Could you check a few things on this model? Use its own coordinates, in mm. Face numbers are marked on the shaded views. Give positions to 0.01 mm unless a question says otherwise; leave off trailing zeros. Loops run counter-clockwise (first coordinate to the right, second up) from the corner with the lowest first, then second, coordinate; pieces in that order, holes last. Notation, with made-up numbers: M 75.25,55.5 L 98.25,55.5 A25 ccw 98.25,72.5 Z; hole C 54.5,80 d4. An arc over 180 degrees is marked long. Write each question's results on one line, items separated by ' | '. Start each with the question number.
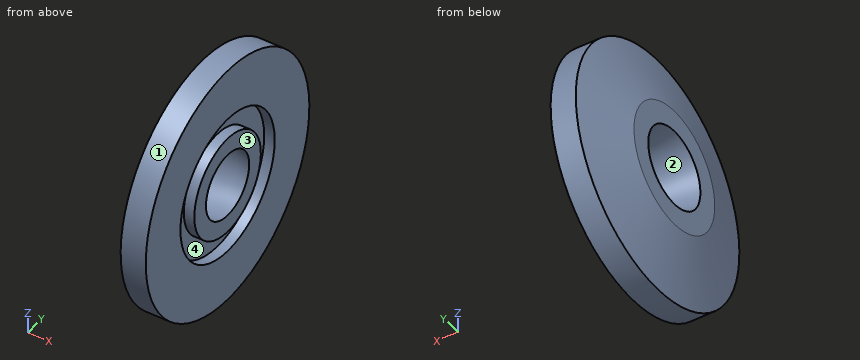
from build123d import *


with BuildPart() as part:
    # Sketch1 → Revolve1 (revolve)
    with BuildSketch(Plane.XY, mode=Mode.PRIVATE) as revolve1_sk:
        Polygon((-2.54, 8.636), (-2.54, 14.986), (-5.588, 14.986), (-7.62, 7.402472759), (-7.62, 0), (-2.54, 0), (-2.54, 6.096), (-3.81, 6.096), (-3.81, 8.636), align=None)
    revolve(revolve1_sk.sketch.rotate(Axis((-12.512764007, 0, 0), (-1, 0, 0)), 90), axis=Axis((-12.512764007, 0, 0), (-1, 0, 0)))

    # Sketch2 → Cut-Revolve1 (revolve, cut)
    with BuildSketch(Plane.XY, mode=Mode.PRIVATE) as cut_revolve1_sk:
        Polygon((-9.728542139, 0), (0.013390026, 0), (0.013390026, 3.553074477), (-9.728542139, 5.111363938), align=None)
    revolve(cut_revolve1_sk.sketch.rotate(Axis((-9.728542139, 0, 0), (-1, 0, 0)), 270), axis=Axis((-9.728542139, 0, 0), (-1, 0, 0)), mode=Mode.SUBTRACT)


solid = part.part
1) Thinking about a two-plate mould opening in Y: for the marked faces 1, 2, 3 and 4, which applies, pulls with the +Y half, pulls with the -Y half, needs draft (parallel to the pull), parting line crosses it, or undercut?
2) If we section it at A-A on y = 0: Write out the boundary of the cut face in (x, z), plus the area to 3 significant figures.
3) If we section it at C-C on x = -6.9: Write out the boundary of the cut face in (y, z).
4) I'm going to push flat-ended pins straight in: P1, Ø1.5, axis at y = -7, z = 1, coming from the +X side; P2, Ø2, axis at y = -8, z = 3, coming from the +X side. Where does each tip first touch, or does it pass through?
5) Please list where these lines run through material, in increasing order: line 1 (Y direction, x = -3.1, z = 0); line 2 (Y direction, x = -3.25, z = 0); line 3 (Y direction, x = -3, z = 4.25). Write a range as from..to.
Calculated:
1) face 1: parting line crosses it | face 2: undercut | face 3: needs draft | face 4: undercut
2) outline: M -7.62,-7.4 L -5.59,-14.99 L -2.54,-14.99 L -2.54,-8.64 L -3.81,-8.64 L -3.81,-6.1 L -2.54,-6.1 L -2.54,-3.96 L -7.62,-4.77 Z; M -7.62,4.77 L -2.54,3.96 L -2.54,6.1 L -3.81,6.1 L -3.81,8.64 L -2.54,8.64 L -2.54,14.99 L -5.59,14.99 L -7.62,7.4 Z | area: 86.0 mm2
3) outline: C 0,0 d20.18; hole C 0,0 d9.32
4) P1: stops at x = -3.81 | P2: stops at x = -2.54
5) line 1: y = -14.99..-8.64, -6.1..-4.05, 4.05..6.1, 8.64..14.99 | line 2: y = -14.99..-8.64, -6.1..-4.08, 4.08..6.1, 8.64..14.99 | line 3: y = -14.37..-7.52, -4.37..4.37, 7.52..14.37
